The listing builds one solid part. Answer for the finished solid, in the listing's coordinates (mm). A direction names the side the tool comes from. Give positions to 0.01 mm unless a question says otherwise; leave off trailing zeros. Order: outer loops, then holes, each group sorted by start corner. A loop starts at its lowest first (then second) coordinate and runs counter-clockwise, first axis right, second up.
```python
from build123d import *

# Parameters (mm, degrees)
F0_W      = 127
F0_H      = 127
F1_DEPTH  = 127
F2_R      = 12.7
F3_DEPTH  = 6.35
F4_R      = 12.7
F5_DEPTH  = 6.35
F6_R      = 12.7
F7_DEPTH  = 6.35
F8_R      = 12.7
F9_DEPTH  = 6.35
F10_R     = 12.7
F11_DEPTH = 6.35
F12_R     = 12.7
F13_DEPTH = 6.35


with BuildPart() as f1:
    # F0 (on Top) → F1 (new body)
    with BuildSketch(Plane.XY):
        with Locations((63.5, 63.5)):
            Rectangle(F0_W, F0_H)
    extrude(amount=F1_DEPTH)

    # F2 (on face) → F3 (cut)
    with BuildSketch(Plane.XY.offset(127)):
        with Locations((63.5, 63.5)):
            Circle(F2_R)
    extrude(amount=-F3_DEPTH, mode=Mode.SUBTRACT)

    # F4 (on face) → F5 (cut)
    with BuildSketch(Plane(origin=(0, 127, 0), x_dir=(-1, 0, 0), z_dir=(0, 1, 0))):
        with Locations((-104.775, 22.225)):
            Circle(F4_R)
        with Locations((-22.225, 104.775)):
            Circle(F4_R)
    extrude(amount=-F5_DEPTH, mode=Mode.SUBTRACT)

    # F6 (on face) → F7 (cut)
    with BuildSketch(Plane(origin=(0, 0, 0), x_dir=(0, -1, 0), z_dir=(-1, 0, 0))):
        with Locations((-104.775, 22.225)):
            Circle(F6_R)
        with Locations((-63.5, 63.5)):
            Circle(F6_R)
        with Locations((-22.225, 104.775)):
            Circle(F6_R)
    extrude(amount=-F7_DEPTH, mode=Mode.SUBTRACT)

    # F8 (on face) → F9 (cut)
    with BuildSketch(Plane.YZ.offset(127)):
        with Locations((22.225, 99.482931)):
            Circle(F8_R)
        with Locations((104.775, 104.775)):
            Circle(F8_R)
        with Locations((104.775, 22.225)):
            Circle(F8_R)
        with Locations((22.225, 22.225)):
            Circle(F8_R)
    extrude(amount=-F9_DEPTH, mode=Mode.SUBTRACT)

    # F10 (on face) → F11 (cut)
    with BuildSketch(Plane.XZ):
        with Locations((104.775, 104.775)):
            Circle(F10_R)
        with Locations((104.775, 22.225)):
            Circle(F10_R)
        with Locations((22.225, 22.225)):
            Circle(F10_R)
        with Locations((63.5, 63.5)):
            Circle(F10_R)
        with Locations((22.225, 104.775)):
            Circle(F10_R)
    extrude(amount=-F11_DEPTH, mode=Mode.SUBTRACT)

    # F12 (on face) → F13 (cut)
    with BuildSketch(Plane(origin=(0, 0, 0), x_dir=(1, 0, 0), z_dir=(0, 0, -1))):
        with Locations((22.225, -22.225)):
            Circle(F12_R)
        with Locations((22.225, -63.5)):
            Circle(F12_R)
        with Locations((22.225, -104.775)):
            Circle(F12_R)
        with Locations((104.775, -22.225)):
            Circle(F12_R)
        with Locations((104.775, -63.5)):
            Circle(F12_R)
        with Locations((104.775, -104.775)):
            Circle(F12_R)
    extrude(amount=-F13_DEPTH, mode=Mode.SUBTRACT)


solid = f1.part
```
1) A tool of negligible diameter and unlimited length cuts with its end or side. For faces 1 (the cylindrical face through (116.89, 59.69, 3.13)), 2 (the flat face through (22, 6.35, 22)), 3 (the flat face through (120.65, 22, 22)), 4 (the flat face through (6.35, 64, 64)), 5 (the cylindrical face through (23.878, 123.869, 117.367)), from which of +Z, -Z, +X, -X, +Y, -Y can it reach the whole face along a straight path? Write none if from no direction.
Geometry says:
face 1: -Z
face 2: -Y
face 3: +X
face 4: -X
face 5: +Y
2) Find section A-A (z = 63.5). Write down the section's boundary in (x, y), then the cut area to 3 significant figures.
Geometry says:
outline: (0, 0) - (50.8, 0) - (50.8, 6.35) - (76.2, 6.35) - (76.2, 0) - (127, 0) - (127, 127) - (0, 127) - (0, 76.2) - (6.35, 76.2) - (6.35, 50.8) - (0, 50.8) - close
area: 15,800 mm2
3) Find section D-D (y = 115). Write down the section's boundary in (x, z), then the cut area to 3 significant figures.
Geometry says:
outline: (0, 0) - (14.69, 0) - (14.69, 6.35) - (29.76, 6.35) - (29.76, 0) - (97.24, 0) - (97.24, 6.35) - (112.31, 6.35) - (112.31, 0) - (127, 0) - (127, 14.69) - (120.65, 14.69) - (120.65, 29.76) - (127, 29.76) - (127, 97.24) - (120.65, 97.24) - (120.65, 112.31) - (127, 112.31) - (127, 127) - (0, 127) - (0, 29.76) - (6.35, 29.76) - (6.35, 14.69) - (0, 14.69) - close
area: 15,700 mm2
4) Given P1, Ø12.5, axis at x = 106.5, y = 65, coming from the -Z side; P2, Ø12.5, axis at x = 104.5, z = 98.5, coming from the -Y side; P3, Ø12.5, axis at y = 19.5, z = 23, coming from the +X side, each flat-ended and moving along its own axis, determine where each tip first touches the part or whether it passes through.
Geometry says:
P1: stops at z = 6.35
P2: stops at y = 6.35
P3: stops at x = 120.65
5) Find section C-C (x = 63.5). Write down the section's boundary in (y, z), then the cut area to 3 significant figures.
Geometry says:
outline: (0, 0) - (127, 0) - (127, 127) - (76.2, 127) - (76.2, 120.65) - (50.8, 120.65) - (50.8, 127) - (0, 127) - (0, 76.2) - (6.35, 76.2) - (6.35, 50.8) - (0, 50.8) - close
area: 15,800 mm2
6) For a pull along Y with two mould halves and no side action, classify faces 6 (the cylindrical face through (20.572, 9.633, 3.131)), 7 (the cylindrical face through (19.472, 3.131, 9.827)), 8 (the flat face through (22, 6.35, 105)) as +Y half, -Y half, draft (parallel to the pull), parting line (faces both ways), or undercut.
Geometry says:
face 6: undercut
face 7: draft
face 8: -Y half
7) Straight lines are drawn through the part: probe 1 along X at (y, z) = (63.5, 3) (3 decimals); probe 2 along X at (y, z) = (25.5, 23); probe 3 along Y at (x, z) = (20, 24.5). For each, find the intervals that lie inside material, in ascending order.
Geometry says:
probe 1: x = 0 to 9.525, 34.925 to 92.075, 117.475 to 127
probe 2: x = 0 to 120.65
probe 3: y = 6.35 to 127
8) Find section B-B (y = 63.5). Write down the section's boundary in (x, z) (3 decimals).
Geometry says:
outline: (0, 0) - (9.525, 0) - (9.525, 6.35) - (34.925, 6.35) - (34.925, 0) - (92.075, 0) - (92.075, 6.35) - (117.475, 6.35) - (117.475, 0) - (127, 0) - (127, 127) - (76.2, 127) - (76.2, 120.65) - (50.8, 120.65) - (50.8, 127) - (0, 127) - (0, 76.2) - (6.35, 76.2) - (6.35, 50.8) - (0, 50.8) - close
